Solid Edge part; units mm, degrees
sketch "Sketch1" plane through (0, 0, 0) normal (0, -1, 0) x (1, 0, 0)
  line L0 (0, 0) -> (14, 0)
  line L1 (14, 0) -> (14, 2)
  line L2 (14, 2) -> (21, 2)
  line L3 (21, 2) -> (21, 8)
  line L4 (21, 8) -> (0, 8)
  dimension "D1" = 21
revolve "RevolvedProtrusion1" add sketch "Sketch1" angle 360 about axis through (0, 0, 10) along (0, 0, -1)
chamfer "Chamfer1" distance 3 angle 45 1 edges at (-21, 0, 8)
hole "Hole_1" at (0, 0, 8) direction (0, 0, -1) diameter 4.8 end up to next countersink diameter 9.18 countersink angle 90
properties material "Polyethylene, low density"
Verification items for the finished model (mm, model axes). A direction names the side the tool comes from. Give positions to 0.01 mm unless a question says otherwise; leave off trailing zeros. Order: outer loops, then holes, each group sorted by start corner. A loop starts at its lowest first (then second) coordinate and runs counter-clockwise, first axis right, second up. Notation, with made-up numbers: M 82.5,83 L 105.5,83 A18 cw 105.5,99 Z; hole C -7.5,40 d11. An arc over 180 degrees is marked long. Answer in a Markdown table with one row per item. Add a question column.
Item 1: Gauge pin test, flat ends, axial feed: pin 1 (1.5 mm diameter, centred on x = -14.5, z = 2, fed in from +Y); pin 2 (3 mm diameter, centred on x = 4, z = 3, fed in from -Y); pin 3 (3 mm diameter, centred on x = 13, y = 12.5, fed in from -Z). Record the tip position at first contact, or that the pin passes through.
Item 2: Tool access check on faces 1 (the cylindrical face through (12.932, -5.362, 1.014)), 2 (the conical face through (-3.94, 17.76, 7.81)). Record the directions out of +Z, -Z, +X, -X, +Y, -Y that give a thin tool (end or side, any length) a straight path to the whole face; none if there is none.
Item 3: Section check C-C, the plane z = 2.75. Enter the section's corners in (x, y).
Item 4: Mould release check, pull along X, two halves, no side actions. Record for faces 3 (the cylindrical face through (2.024, -1.29, 2.946)), 4 (the cylindrical face through (20.03, 6.31, 3.52)), 5 (the flat face through (4, 4, 8)): released by +X, released by -X, zero draft, split by the parting line, or undercut.
Item 5: Section check A-A, the plane y = 0. Enter the section's corners in (x, z).
Item 6: Scan lines: probe 1 along X at (y, z) = (0, 3.55); probe 2 along X at (y, z) = (-2, 3.25). Record each from-to range of solid material in increasing order. Write a range as from..to.
Filled sheet:
| question | item | result |
|---|---|---|
| 1 | pin 1 | stops at y = 15.87 |
| 1 | pin 2 | stops at y = -20.85 |
| 1 | pin 3 | stops at z = 2 |
| 2 | face 1 | -Z |
| 2 | face 2 | +Z |
| 3 | outline | C 0,0 d42; hole C 0,0 d4.8 |
| 4 | face 3 | undercut |
| 4 | face 4 | split by the parting line |
| 4 | face 5 | zero draft |
| 5 | outline | M -21,2 L -14,2 L -14,0 L -2.4,0 L -2.4,5.81 L -4.59,8 L -18,8 L -21,5 Z; M 2.4,0 L 14,0 L 14,2 L 21,2 L 21,5 L 18,8 L 4.59,8 L 2.4,5.81 Z |
| 6 | probe 1 | x = -21..-2.4, 2.4..21 |
| 6 | probe 2 | x = -20.9..-1.33, 1.33..20.9 |
